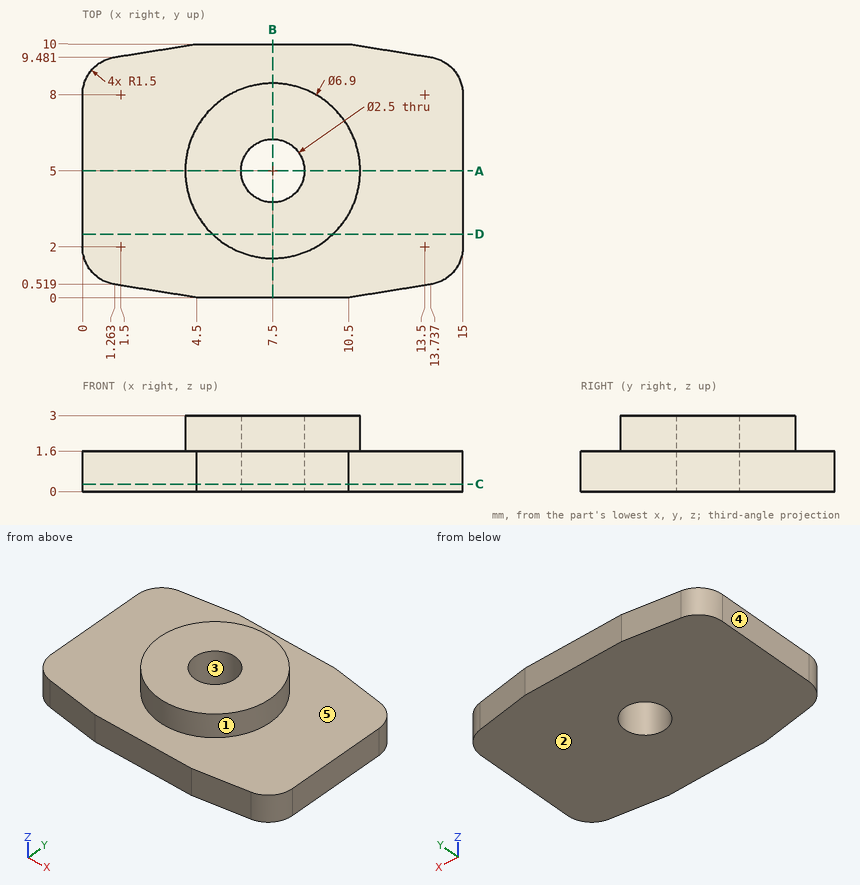
The drawing under review shows one solid part. Ordinate dimensions are in mm from its lowest x, y, z. A direction names the side the tool comes from. Round coordinates to 2 decimals unless told otherwise and drop trailing zeros. Order: outer loops, then holes, each group sorted by start corner. A loop starts at its lowest first (then second) coordinate and runs counter-clockwise, first axis right, second up. Notation, with made-up numbers: (33.5, 23) -> (66.5, 23) arc R25 cw to (66.5, 50) -> close; hole circle Ø4 at (25.5, -7.5). An arc over 180 degrees is marked (long way). Return JSON: item names as keys, results as strings.
1. For L1, parallel to Y at x = 7.5, z = 0.8; L2, parallel to Y at x = 7.5, z = 2.2; L3, parallel to Z at x = 6.25, y = 1.25, list the stretches that pass through material, from the lowest coordinate up. Write a range as [from, to].
Answer block:
{"L1": "y = [0, 3.75], [6.25, 10]", "L2": "y = [1.55, 3.75], [6.25, 8.45]", "L3": "z = [0, 1.6]"}
2. Take a section at A-A (y = 5). Write out the cut boundary in (x, z).
Answer block:
{"outline": "(0, 0) -> (6.25, 0) -> (6.25, 3) -> (4.05, 3) -> (4.05, 1.6) -> (0, 1.6) -> close; (8.75, 0) -> (15, 0) -> (15, 1.6) -> (10.95, 1.6) -> (10.95, 3) -> (8.75, 3) -> close"}
3. The part is to be moulded in two halves that separate along X. For the marked faces 3, 4 and 5, say which applies: +X half, -X half, draft (parallel to the pull), parting line (faces both ways), or undercut.
Answer block:
{"face 3": "undercut", "face 4": "-X half", "face 5": "draft"}
4. For the marked faces 1 and 2, list the 3-axis set-ups (+Z, -Z, +X, -X, +Y, -Y) from which the entire face can be reached by the end or side of a thin tool; tool diameter is ignored.
Answer block:
{"face 1": "+Z", "face 2": "-Z, +X, -X, +Y, -Y"}
5. Take a section at D-D (y = 2.5). Write out the cut boundary in (x, z).
Answer block:
{"outline": "(0, 0) -> (15, 0) -> (15, 1.6) -> (9.88, 1.6) -> (9.88, 3) -> (5.12, 3) -> (5.12, 1.6) -> (0, 1.6) -> close"}
6. Take a section at C-C (z = 0.3). Write out the cut boundary in (x, y).
Answer block:
{"outline": "(0, 2) arc R1.5 ccw to (1.26, 0.52) -> (4.5, 0) -> (10.5, 0) -> (13.74, 0.52) arc R1.5 ccw to (15, 2) -> (15, 8) arc R1.5 ccw to (13.74, 9.48) -> (10.5, 10) -> (4.5, 10) -> (1.26, 9.48) arc R1.5 ccw to (0, 8) -> close; hole circle Ø2.5 at (7.5, 5)"}
7. Take a section at B-B (x = 7.5). Write out the cut boundary in (y, z).
Answer block:
{"outline": "(0, 0) -> (3.75, 0) -> (3.75, 3) -> (1.55, 3) -> (1.55, 1.6) -> (0, 1.6) -> close; (6.25, 0) -> (10, 0) -> (10, 1.6) -> (8.45, 1.6) -> (8.45, 3) -> (6.25, 3) -> close"}
